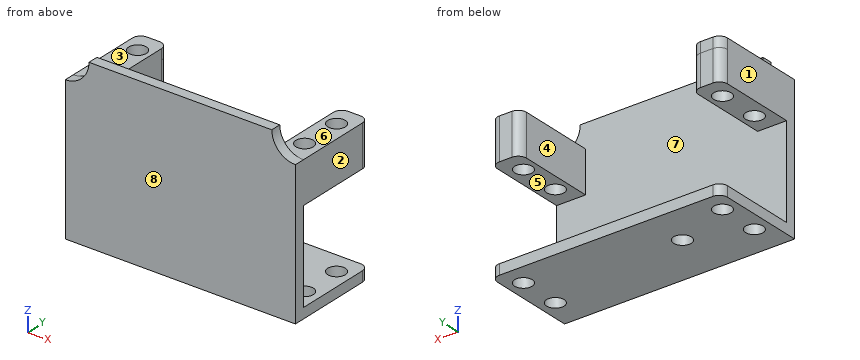
```python
from build123d import *

# Parameters (mm, degrees)
SKETCH1_W                   = 55.5
SKETCH1_H                   = 37.9
BRACKETBASE_DEPTH           = 2.5
SKETCH2_W                   = 7
SKETCH2_H                   = 20.5
SERVOMOUNTINGHOLETABS_DEPTH = 2.5
SKETCH3_R                   = 2.125
SERVOMOUNTINGHOLES_DEPTH    = 2.5
SKETCH4_W                   = 55.5
SKETCH4_H                   = 2.5
BASEWALL_DEPTH              = 23
SKETCH6_R                   = 5.7
BASETRIM_DEPTH              = 2.5
FILLET1_R                   = 2
SKETCH7_R                   = 2.125
M4MOUNTINGHOLE_DEPTH        = 10
SKETCH8_R                   = 2.125
BOSS_EXTRUDE1_DEPTH         = 7.5
SKETCH9_R                   = 2.125
CUT_EXTRUDE1_DEPTH          = 70.378238663


with BuildPart() as part:
    # Sketch1 → bracketBase (new body)
    with BuildSketch(Plane(origin=(0, 0, 0), x_dir=(1, 0, 0), z_dir=(0, 1, 0))):
        with Locations((27.75, 18.95)):
            Rectangle(SKETCH1_W, SKETCH1_H)
    extrude(amount=BRACKETBASE_DEPTH)

    # Sketch2 → servoMountingHoleTabs (add)
    with BuildSketch(Plane.XY.offset(-8.2)):
        with Locations((3.5, 12.75)):
            Rectangle(SKETCH2_W, SKETCH2_H)
        with Locations((52, 12.75)):
            Rectangle(SKETCH2_W, SKETCH2_H)
    extrude(amount=SERVOMOUNTINGHOLETABS_DEPTH)

    # Sketch3 → servoMountingHoles (cut)
    with BuildSketch(Plane.XY.offset(-5.7)):
        with Locations((3.75, 17.75)):
            Circle(SKETCH3_R)
        with Locations(Location((3.75, 7.75, 0), (0, 0, 180))):
            Circle(SKETCH3_R)
        with Locations((51.75, 7.75)):
            Circle(SKETCH3_R)
        with Locations(Location((51.75, 17.75, 0), (0, 0, 180))):
            Circle(SKETCH3_R)
    extrude(amount=-SERVOMOUNTINGHOLES_DEPTH, mode=Mode.SUBTRACT)

    # Sketch4 → baseWall (add)
    with BuildSketch(Plane(origin=(0, 0, 0), x_dir=(1, 0, 0), z_dir=(0, 1, 0))):
        with Locations((27.75, 39.15)):
            Rectangle(SKETCH4_W, SKETCH4_H)
    extrude(amount=BASEWALL_DEPTH)

    # Sketch6 → baseTrim (cut)
    with BuildSketch(Plane(origin=(0, 2.5, 0), x_dir=(1, 0, 0), z_dir=(0, 1, 0))):
        Circle(SKETCH6_R)
        with Locations((55.5, 0)):
            Circle(SKETCH6_R)
    extrude(amount=-BASETRIM_DEPTH, mode=Mode.SUBTRACT)

    # Fillet1
    fillet1_edges = [part.edges().sort_by_distance(p)[0] for p in [
        (0, 23, -6.95),
        (7, 23, -6.95),
        (55.5, 23, -6.95),
        (48.5, 23, -6.95),
        (55.5, 23, -39.15),
        (0, 23, -39.15),
    ]]
    fillet(fillet1_edges, radius=FILLET1_R)

    # Sketch7 → M4mountingHole (cut)
    with BuildSketch(Plane(origin=(0, 0, -40.4), x_dir=(-1, 0, 0), z_dir=(0, 0, -1))):
        with Locations((-17.25, 12.75)):
            Circle(SKETCH7_R)
    extrude(amount=-M4MOUNTINGHOLE_DEPTH, mode=Mode.SUBTRACT)

    # Sketch8 → Boss-Extrude1 (add)
    # profile 1 of 2: a face of its own
    with BuildSketch(Plane(origin=(0, 0, -8.2), x_dir=(-1, 0, 0), z_dir=(0, 0, -1))):
        with BuildLine():
            Line((-48.5, 2.5), (-48.5, 21))
            ThreePointArc((-48.5, 21), (-49.085786438, 22.414213562), (-50.5, 23))
            Line((-50.5, 23), (-53.5, 23))
            ThreePointArc((-53.5, 23), (-54.914213562, 22.414213562), (-55.5, 21))
            Line((-55.5, 21), (-55.5, 2.5))
            Line((-55.5, 2.5), (-48.5, 2.5))
        make_face()
        with Locations((-51.75, 17.75)):
            Circle(SKETCH8_R, mode=Mode.SUBTRACT)
        with Locations(Location((-51.75, 7.75, 0), (0, 0, 180))):
            Circle(SKETCH8_R, mode=Mode.SUBTRACT)
    # profile 2 of 2: a face of its own
    with BuildSketch(Plane(origin=(0, 0, -8.2), x_dir=(-1, 0, 0), z_dir=(0, 0, -1))):
        with BuildLine():
            Line((-2, 23), (-5, 23))
            ThreePointArc((-5, 23), (-6.414213562, 22.414213562), (-7, 21))
            Line((-7, 21), (-7, 2.5))
            Line((-7, 2.5), (0, 2.5))
            Line((0, 2.5), (0, 21))
            ThreePointArc((0, 21), (-0.585786438, 22.414213562), (-2, 23))
        make_face()
        with Locations(Location((-3.75, 17.75, 0), (0, 0, 180))):
            Circle(SKETCH8_R, mode=Mode.SUBTRACT)
        with Locations((-3.75, 7.75)):
            Circle(SKETCH8_R, mode=Mode.SUBTRACT)
    extrude(amount=BOSS_EXTRUDE1_DEPTH)

    # Sketch9 → Cut-Extrude1 (cut, through all)
    with BuildSketch(Plane.XY.offset(-5.7)):
        with Locations((3.75, 17.75)):
            Circle(SKETCH9_R)
        with Locations(Location((3.75, 7.75, 0), (0, 0, 180))):
            Circle(SKETCH9_R)
        with Locations(Location((51.75, 17.75, 0), (0, 0, 180))):
            Circle(SKETCH9_R)
        with Locations((51.75, 7.75)):
            Circle(SKETCH9_R)
    extrude(amount=-CUT_EXTRUDE1_DEPTH, mode=Mode.SUBTRACT)


solid = part.part
```
Check sheet for the modelled part. Datum: model origin and axes. Units: mm. Face numbers are marked on the shaded views. A direction names the side the tool comes from. Round coordinates to 2 decimals unless told otherwise and drop trailing zeros. Order: outer loops, then holes, each group sorted by start corner. A loop starts at its lowest first (then second) coordinate and runs counter-clockwise, first axis right, second up.
1) Go/stop test with flat-tipped pins: pin 1 Ø7 at (x, y) = (51.75, 17.75) entering from +Z; pin 2 Ø1.5 at (x, z) = (34.5, -10) entering from +Y; pin 3 Ø3.5 at (x, y) = (3.75, 7.75) entering from -Z; pin 4 Ø1 at (x, y) = (23, 18.5) entering from +Z. Record where each tip stops, or that it passes through.
2) Scan lines: line 1 (X direction, y = 7.75, z = -13.5) (3 decimals); line 2 (Y direction, x = 3.75, z = -6.15) (3 decimals); line 3 (Z direction, x = 50, y = 14.25). Record each from-to range of solid material in increasing order.
3) Section check D-D (y = 12.75). Record the boundary of the cut face in (x, z) (3 decimals), and give its area (3 significant figures).
4) Section check C-C (y = 5). Record the boundary of the cut face in (x, z), and give its area (3 significant figures).
5) Section check B-B (x = 17.25). Record the boundary of the cut face in (y, z) (3 decimals), and give its area (3 significant figures).
6) Tool access check on the marked faces 1, 2, 3, 4 and 5. Record the directions out of +Z, -Z, +X, -X, +Y, -Y that give a thin tool (end or side, any length) a straight path to the whole face; none if there is none.
7) Section check A-A (z = -12.5). Record the boundary of the cut face in (x, y) (3 decimals).
8) Mould release check, pull along Z, two halves, no side actions. Record for the marked faces 6, 7 and 8: +Z half, -Z half, draft (parallel to the pull), parting line (faces both ways), or undercut.
Result:
1. pin 1: stops at z = -5.7
1. pin 2: stops at y = 2.5
1. pin 3: passes through
1. pin 4: stops at z = -37.9
2. line 1: x = 0 to 1.625, 5.875 to 7, 48.5 to 49.625, 53.875 to 55.5
2. line 2: y = 0 to 5.625, 9.875 to 15.625, 19.875 to 23
2. line 3: z = -40.4 to -37.9, -15.7 to -5.7
3. outline: (0, -40.4) - (15.125, -40.4) - (15.125, -37.9) - (0, -37.9) - close; (0, -15.7) - (7, -15.7) - (7, -5.7) - (0, -5.7) - close; (19.375, -40.4) - (55.5, -40.4) - (55.5, -37.9) - (19.375, -37.9) - close; (48.5, -15.7) - (55.5, -15.7) - (55.5, -5.7) - (48.5, -5.7) - close
3. area: 268 mm2
4. outline: (0, -40.4) - (55.5, -40.4) - (55.5, -37.9) - (0, -37.9) - close; (0, -15.7) - (7, -15.7) - (7, -5.7) - (0, -5.7) - close; (48.5, -15.7) - (55.5, -15.7) - (55.5, -5.7) - (48.5, -5.7) - close
4. area: 279 mm2
5. outline: (0, -40.4) - (10.625, -40.4) - (10.625, -37.9) - (2.5, -37.9) - (2.5, 0) - (0, 0) - close; (14.875, -40.4) - (23, -40.4) - (23, -37.9) - (14.875, -37.9) - close
5. area: 142 mm2
6. face 1: +Z, -Z, -X, +Y, -Y
6. face 2: +Z, -Z, +X, +Y, -Y
6. face 3: +Z, +X, -X, +Y
6. face 4: +Z, +Y
6. face 5: +X, -X, +Y
7. outline: (0, 0) - (55.5, 0) - (55.5, 21) arc R2 ccw to (53.5, 23) - (50.5, 23) arc R2 ccw to (48.5, 21) - (48.5, 2.5) - (7, 2.5) - (7, 21) arc R2 ccw to (5, 23) - (2, 23) arc R2 ccw to (0, 21) - close; hole circle Ø4.25 at (3.75, 7.75); hole circle Ø4.25 at (3.75, 17.75); hole circle Ø4.25 at (51.75, 7.75); hole circle Ø4.25 at (51.75, 17.75)
8. face 6: +Z half
8. face 7: undercut
8. face 8: draft
